Part model, mm, in its own coordinate system. Coordinates: 2 decimals unless noted, no trailing zeros. Write each loop counter-clockwise with the first axis right and the second up, starting at its lowest first coordinate (ties: lowest second). Pieces come first, ordered by that corner, then holes. Notation, with made-up numbers: (62, -32.75) -> (109, -32.75) arc R21 ccw to (109, 0.25) -> close; hole circle Ø1 at (50, 67.5). An arc over 180 degrees is marked (long way). Write item = value, one per line.
Autodesk Inventor part; units mm, degrees
ref_plane "YZ Plane" through (0, 0, 0) normal (1, 0, 0) x (0, 1, 0)
ref_plane "XZ Plane" through (0, 0, 0) normal (0, 1, 0) x (-1, 0, 0)
ref_plane "XY Plane" through (0, 0, 0) normal (0, 0, 1) x (1, 0, 0)
sketch "Sketch1" plane through (0, 0, 0) normal (0, 1, 0) x (-1, 0, 0)
  circle A0 centre (0, 0) radius 139.7
  circle A1 centre (107.2204, 62.9369) radius 1.5875
  circle A2 centre (-107.2204, 62.9369) radius 1.5875
  circle A3 centre (107.2204, -62.9369) radius 1.5875
  circle A4 centre (-107.2204, -62.9369) radius 1.5875
  circle A5 centre (73.2444, -95.6484) radius 1.5875
  circle A6 centre (73.2444, -0.3984) radius 1.5875
  circle A7 centre (-73.025, -0.3984) radius 1.5875
  circle A8 centre (-72.8056, -95.6484) radius 1.5875
  ellipse E0 centre (0.4389, -48.0234) end of major axis (-72.5861, -48.0234) minor radius 47.625
  circle A9 centre (0, 133.35) radius 1.5875
  circle A10 centre (-133.35, 0) radius 1.5875
  circle A11 centre (0, -133.35) radius 1.5875
  circle A12 centre (133.35, 0) radius 1.5875
  circle A13 centre (-25.4, 117.8713) radius 6.35
  circle A14 centre (25.4, 117.8713) radius 3.175
  circle A15 centre (-83.3566, 29.2053) radius 1.5875
  circle A16 centre (-41.7006, 29.2053) radius 1.5875
  circle A17 centre (-41.7006, 96.5153) radius 1.5875
  circle A18 centre (-83.3566, 96.5153) radius 1.5875
  ellipse E1 centre (-62.5286, 62.8603) end of major axis (-62.5286, 29.2053) minor radius 20.828
  circle A19 centre (6.25, 127) radius 1.1303
  circle A20 centre (-6.25, 127) radius 1.1303
  circle A21 centre (-127, -6.25) radius 1.1303
  circle A22 centre (-127, 6.25) radius 1.1303
  circle A23 centre (6.25, -127) radius 1.1303
  circle A24 centre (-6.25, -127) radius 1.1303
  circle A25 centre (127, 6.25) radius 1.1303
  circle A26 centre (127, -6.25) radius 1.1303
  circle A27 centre (0, 42.9864) radius 12.7
  circle A28 centre (41.7006, 29.2053) radius 1.5875
  circle A29 centre (83.3566, 29.2053) radius 1.5875
  ellipse E2 centre (62.5286, 62.8603) end of major axis (62.5286, 29.2053) minor radius 20.828
  circle A30 centre (41.7006, 96.5153) radius 1.5875
  circle A31 centre (83.3566, 96.5153) radius 1.5875
  dimension "d0" = 279.4
  dimension "d60" = 3.175
  dimension "d92" = 3.175
  dimension "d93" = 3.175
  dimension "d94" = 3.175
  dimension "d95" = 3.175
  dimension "d97" = 3.175
  dimension "d100" = 360
  dimension "d102" = 12.7
  dimension "d103" = 6.35
  dimension "d118" = 2.2606
  dimension "d121" = 50.8
  dimension "d122" = 25.4
  dimension "d123" = 25.4
  dimension "d125" = 73.025
  dimension "d126" = 146.05
extrude "Extrusion9" add sketch "Sketch1" along normal blind 6.35
properties part number "Base_Acryllic"
Q1. Pin check, flat tips, straight feed: pin 1 (1.4 mm diameter, centred on x = 6.25, z = 127, fed in from -Y); pin 2 (1.5 mm diameter, centred on x = 26.5, y = 4, fed in from -Z); pin 3 (3 mm diameter, centred on x = 58, y = 1, fed in from +Z). Stop position of each tip, or through.
Model answer:
pin_1 = through
pin_2 = -137.31
pin_3 = 127.76
Q2. Probe line 1 (Z direction, x = 0, y = 3); line 2 (Z direction, x = -6.25, y = 4); line 3 (Z direction, x = 11.5, y = 6). List the from-to ranges inside material, lowest first. Write a range as from..to.
Model answer:
line_1 = -139.7..-134.94, -131.76..-95.65, -0.4..30.29, 55.69..131.76, 134.94..139.7
line_2 = -139.56..-128.13, -125.87..-95.5, -0.55..31.93, 54.04..125.87, 128.13..139.56
line_3 = -139.23..-95.01, -1.04..37.6, 48.38..139.23
Q3. Saw through at A-A on x = 47. Count the separate pieces of the cut face and the enclosed holes in it, and give its area (3 significant figures).
Model answer:
separate_pieces = 3
enclosed_holes = 0
area = 926 mm²
Q4. Saw through at D-D on x = -96. Give the cut face in (y, z), and give its area (3 significant figures).
Model answer:
outline = (0, -101.49) -> (6.35, -101.49) -> (6.35, 101.49) -> (0, 101.49) -> close
area = 1,290 mm²
Q5. Mould opens along X. For faces 1 (the face through (2, 0, 2)), 2 (the face through (110.86, 3.13, 85.01)), 3 (the face through (1.7, 3.1, 30.4)) say: released by +X, released by -X, zero draft, split by the parting line, or undercut.
Model answer:
face_1 = zero draft
face_2 = split by the parting line
face_3 = undercut
